The drawing under review shows one solid part. Ordinate dimensions are in mm from its lowest x, y, z. A direction names the side the tool comes from. Give positions to 0.01 mm unless a question says otherwise; leave off trailing zeros. Write each loop counter-clockwise with the first axis right and the second up, starting at its lowest first coordinate (ties: lowest second). Pieces come first, ordered by that corner, then holes. Notation, with made-up numbers: M -18,86.25 L 15,86.25 A23 ccw 15,101.25 Z; hole C 10,-25.5 d10. An arc over 180 degrees is marked long. Answer as a JSON object with one key per item and string values. Group by question number.
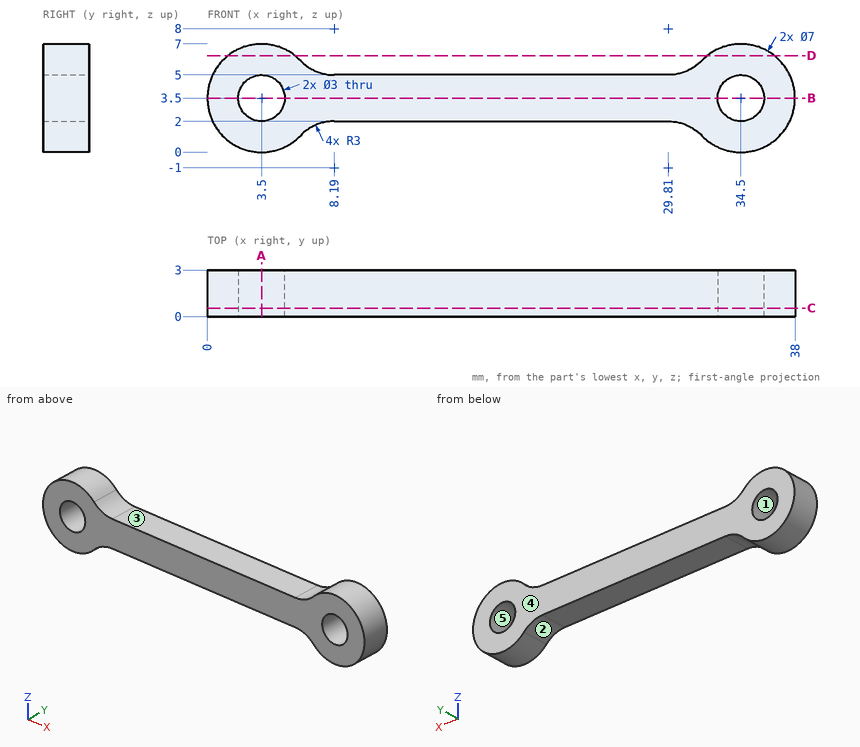
Item 1: Consider section C-C (y = 0.55). Give the boundary of the cut face in (x, z) (1 decimal), plus the area to 3 significant figures.
Item 2: Consider section A-A (x = 3.5). Give the boundary of the cut face in (y, z), plus the area to 3 significant figures.
Item 3: Insertion check: P1, Ø1.5, axis at x = 21, y = 2, coming from the -Z side; P2, Ø2.5, axis at x = 3.5, z = 3.5, coming from the +Y side; P3, Ø1, axis at y = 1, z = 5, coming from the -X side. Each pin has a flat end and moves straight along its axis. Give the tip position at first contact, or say it passes through.
Item 4: Draft analysis for pull direction X (two halves, no side actions). For the marked faces 4 and 5, state which applies: released by +X, released by -X, zero draft, split by the parting line, or undercut.
Item 5: Consider section B-B (z = 3.5). Give the boundary of the cut face in (x, y).
Item 6: To check wall thickness, follow probe 1 along X at (y, z) = (2.05, 3.5); probe 2 along Z at (x, y) = (3.5, 1.75); probe 3 along X at (y, z) = (2.35, 4.25). State the ranges of each line that lie inside material, in increasing order.
Item 7: Machinability: for the marked faces 1, 2 and 3, which of the approach directions +Z, -Z, +X, -X, +Y, -Y give a long, thin tool a straight path to every point of the face, cutting with its end or side? Answer none if there is none.
Item 8: Consider section D-D (z = 6.25). Give the boundary of the cut face in (x, y) (1 decimal).
Result set:
{
 "1": {"outline": "M 6,1.1 A3 cw 8.2,2 L 29.8,2 A3 cw 32,1.1 A3.5 ccw long 32,5.9 A3 cw 29.8,5 L 8.2,5 A3 cw 6,5.9 A3.5 ccw long Z; hole C 3.5,3.5 d3; hole C 34.5,3.5 d3", "area": "137 mm^2"},
 "2": {"outline": "M 0,0 L 3,0 L 3,2 L 0,2 Z; M 0,5 L 3,5 L 3,7 L 0,7 Z", "area": "12.0 mm^2"},
 "3": {"P1": "stops at z = 2", "P2": "passes through", "P3": "stops at x = 0.15"},
 "4": {"face 4": "zero draft", "face 5": "undercut"},
 "5": {"outline": "M 0,0 L 2,0 L 2,3 L 0,3 Z; M 5,0 L 33,0 L 33,3 L 5,3 Z; M 36,0 L 38,0 L 38,3 L 36,3 Z"},
 "6": {"probe 1": "x = 0 to 2, 5 to 33, 36 to 38", "probe 2": "z = 0 to 2, 5 to 7", "probe 3": "x = 0.08 to 2.2, 4.8 to 33.2, 35.8 to 37.92"},
 "7": {"face 1": "+Y, -Y", "face 2": "-Z, +Y, -Y", "face 3": "+Z, +Y, -Y"},
 "8": {"outline": "M 1.3,0 L 5.7,0 L 5.7,3 L 1.3,3 Z; M 32.3,0 L 36.7,0 L 36.7,3 L 32.3,3 Z"}
}
